Design review of the part built by this model. Coordinates are the model's own, in mm. Round coordinates to 2 decimals unless told otherwise and drop trailing zeros. Loops run counter-clockwise (first coordinate to the right, second up) from the corner with the lowest first, then second, coordinate; pieces in that order, holes last. Notation, with made-up numbers: (66.5, 32.25) - (110.5, 32.25) arc R15 ccw to (110.5, 48.25) - close; hole circle Ø10 at (87, -16.75). An arc over 180 degrees is marked (long way). Return JSON: item names as keys, results as strings. Group by question number.
Autodesk Fusion 360 part; units mm, degrees
sketch "Sketch1" plane through (0, 0, 0) normal (0, 0, 1) x (1, 0, 0)
  line L0 (21, -22.5) -> (-21, -22.5)
  line L1 (-21, -22.5) -> (-21, 22.5)
  line L2 (-21, 22.5) -> (21, 22.5)
  line L3 (21, 22.5) -> (21, -22.5)
  line L4 (21, -22.5) -> (-21, 22.5) construction
  line L5 (-21, -22.5) -> (21, 22.5) construction
  line L6 (0, 22.5) -> (0, -22.5)
  line L7 (-21, 0) -> (21, 0)
  line L8 (17.6, 19) -> (17.6, 7)
  line L9 (17.6, -7.9) -> (17.6, -19.9)
  line L10 (11.8, 19) -> (11.8, 7)
  line L11 (11.8, -7.9) -> (11.8, -19.9)
  line L12 (-11.8, 19) -> (-11.8, 7)
  line L13 (-11.8, -7.9) -> (-11.8, -19.9)
  line L14 (-17.6, 19) -> (-17.6, 7)
  line L15 (-17.6, -7.9) -> (-17.6, -19.9)
  line L16 (-17.7333, 19) -> (-11.8, 19)
  line L17 (11.8, 19) -> (17.7333, 19)
  line L18 (-17.6, 7) -> (-11.8, 7)
  line L19 (11.8, 7) -> (17.6, 7)
  line L20 (-17.6, -7.9) -> (-11.8, -7.9)
  line L21 (11.8, -7.9) -> (17.6, -7.9)
  line L22 (-17.6, -19.9) -> (-11.8, -19.9)
  line L23 (11.8, -19.9) -> (17.6, -19.9)
  dimension "d1" = 42
  dimension "d2" = 45
  dimension "d5" = 3.5
  dimension "d6" = 15.5
  dimension "d7" = 30.4
  dimension "d8" = 42.4
extrude "Extrude1" add sketch "Sketch1" along normal blind 3
fillet "Fillet1" radius 2 4 edges at (-21, 22.5, 1.5) (21, 22.5, 1.5) (21, -22.5, 1.5) (-21, -22.5, 1.5)
fillet "Fillet2" radius 2 4 edges at (17.6, 7, 1.5) (11.8, 7, 1.5) (11.8, 19, 1.5) (17.6, 19, 1.5)
fillet "Fillet3" radius 2 4 edges at (-17.6, 19, 1.5) (-11.8, 19, 1.5) (-11.8, 7, 1.5) (-17.6, 7, 1.5)
fillet "Fillet4" radius 2 4 edges at (-11.8, -19.9, 1.5) (-17.6, -19.9, 1.5) (-17.6, -7.9, 1.5) (-11.8, -7.9, 1.5)
fillet "Fillet5" radius 2 4 edges at (11.8, -7.9, 1.5) (17.6, -7.9, 1.5) (11.8, -19.9, 1.5) (17.6, -19.9, 1.5)
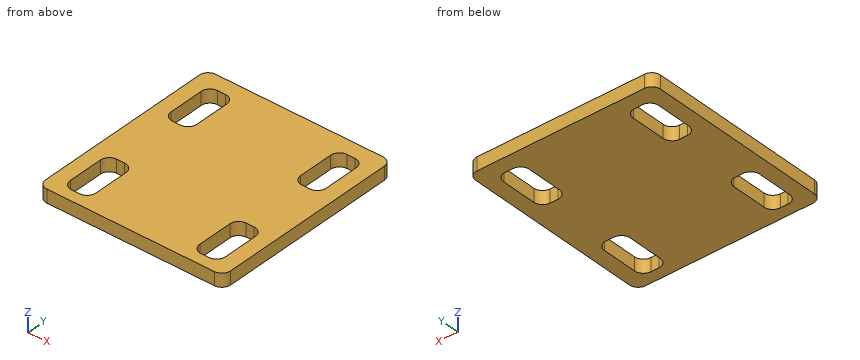
Q1. Add section B-B, the plane z = 1.5. Give the number of separate pieces and of enclosed holes in the cut face, plus the area to 3 significant figures.
Q2. For line 1 (X direction, y = 13.5, z = 2.8); line 2 (Y direction, x = -15, z = 1.3); line 3 (X direction, y = -19, z = 2.5), list the stretches that pass through material, from the lowest coordinate up.
Q3. Add section A-A, the plane y = 11. State the section outline as (x, z) points, plus the area to 3 significant figures.
Q4. Add section C-C, the plane y = -8.5. State the section outline as (x, z) points, plus the area to 3 significant figures.
Evaluation:
{
 "1": {"separate pieces": "1", "enclosed holes": "4", "area": "1,620 mm²"},
 "2": {"line 1": "-21 to -17.6, -11.8 to 11.8, 17.6 to 21", "line 2": "-22.5 to -19.9, -7.9 to 7, 19 to 22.5", "line 3": "-21 to -17.27, -12.13 to 12.13, 17.27 to 21"},
 "3": {"outline": "(-21, 0) - (-17.6, 0) - (-17.6, 3) - (-21, 3) - close; (-11.8, 0) - (11.8, 0) - (11.8, 3) - (-11.8, 3) - close; (17.6, 0) - (21, 0) - (21, 3) - (17.6, 3) - close", "area": "91.2 mm²"},
 "4": {"outline": "(-21, 0) - (-17.03, 0) - (-17.03, 3) - (-21, 3) - close; (-12.37, 0) - (12.37, 0) - (12.37, 3) - (-12.37, 3) - close; (17.03, 0) - (21, 0) - (21, 3) - (17.03, 3) - close", "area": "98.1 mm²"}
}
